Check sheet for the modelled part. Datum: model origin and axes. Units: mm. A direction names the side the tool comes from. Round coordinates to 2 decimals unless told otherwise and drop trailing zeros. Order: outer loops, then holes, each group sorted by start corner. A loop starts at its lowest first (then second) coordinate and runs counter-clockwise, first axis right, second up.
(1) Sectioned sample at C-C, the plane y = 10.5. Enter the section's corners in (x, z), and give its area (3 significant figures).
(2) Sectioned sample at A-A, the plane x = -150. Enter the section's corners in (y, z), and give its area (3 significant figures).
(3) Depth check by flat-ended pin: pin 1 (1.5 mm diameter, centred on x = -39.5, y = 13, fed in from -Z); pin 2 (3 mm diameter, centred on y = 47, z = -23.5, fed in from -X); pin 3 (2 mm diameter, centred on x = -1.5, y = 14, fed in from +Z). Enter the tip coordinate at first touch or a pass-through.
(4) Thickness scan on probe 1 along X at (y, z) = (26, 0); probe 2 along X at (y, z) = (39, 8.5); probe 3 along Y at (x, z) = (126.5, -25). Record the ranges inside material, lowest first.
(5) Sectioned sample at B-B, the plane z = 0. Enter the section's corners in (x, y), and give its area (3 significant figures).
(6) Mould release check, pull along Z, two halves, no side actions. Record for faces 6 (the cylindrical face through (15.02, 34.51, 47.69)), 7 (the cylindrical face through (90.44, 9.86, 36.97)), 8 (the flat face through (45, 70, -23)): released by +Z, released by -Z, zero draft, split by the parting line, or undercut.
(7) Sectioned sample at D-D, the plane x = 0. Enter the section's corners in (y, z), and give its area (3 significant figures).
(8) Tool access check on faces 1 (the cylindrical face through (-91.77, 9.86, 36.69)), 2 (the flat face through (163, 40, -22)), 3 (the flat face through (-138.447, 40, 22.344)), 4 (the cylindrical face through (-90.44, 9.86, -36.97)), 5 (the flat face through (-33, 20, -51)). Record the directions out of +Z, -Z, +X, -X, +Y, -Y that give a thin tool (end or side, any length) a straight path to the whole face; none if there is none.
```python
from build123d import *
from build123d.topology import SkipClean

# Parameters (mm, degrees)
SKETCH1_R           = 60
SKETCH1_R_2         = 25
BOSS_EXTRUDE2_DEPTH = 20
SKETCH1_7_R         = 60
SKETCH1_7_R_2       = 50
BOSS_EXTRUDE3_DEPTH = 70
SKETCH3_R           = 40
SKETCH3_R_2         = 25
BOSS_EXTRUDE4_DEPTH = 20


with BuildPart() as part:
    # Sketch1 → Boss-Extrude2 (new body)
    with BuildSketch(Plane(origin=(0, 0, 0), x_dir=(1, 0, 0), z_dir=(0, 1, 0))):
        with BuildLine():
            ThreePointArc((-139.071428571, 38.478127898), (-190, 0), (-139.071428571, -38.478127898))
            ThreePointArc((-139.071428571, -38.478127898), (-91.104177178, -36.827906099), (-47.892857143, -57.717191847))
            ThreePointArc((-47.892857143, -57.717191847), (0, -75), (47.892857143, -57.717191847))
            ThreePointArc((47.892857143, -57.717191847), (91.104177178, -36.827906099), (139.071428571, -38.478127898))
            ThreePointArc((139.071428571, -38.478127898), (190, 0), (139.071428571, 38.478127898))
            ThreePointArc((139.071428571, 38.478127898), (91.104177178, 36.827906099), (47.892857143, 57.717191847))
            ThreePointArc((47.892857143, 57.717191847), (0, 75), (-47.892857143, 57.717191847))
            ThreePointArc((-47.892857143, 57.717191847), (-91.104177178, 36.827906099), (-139.071428571, 38.478127898))
        make_face()
        with Locations(Location((0, 0, 0), (0, 0, 270))):
            Circle(SKETCH1_R, mode=Mode.SUBTRACT)
        with Locations(Location((-150, 0, 0), (0, 0, 270))):
            Circle(SKETCH1_R_2, mode=Mode.SUBTRACT)
        with Locations(Location((150, 0, 0), (0, 0, 90))):
            Circle(SKETCH1_R_2, mode=Mode.SUBTRACT)
    extrude(amount=BOSS_EXTRUDE2_DEPTH)

    # Sketch1_7 → Boss-Extrude3 (add)
    with BuildSketch(Plane(origin=(0, 0, 0), x_dir=(1, 0, 0), z_dir=(0, 1, 0))):
        with Locations(Location((0, 0, 0), (0, 0, 270))):
            Circle(SKETCH1_7_R)
        with Locations(Location((0, 0, 0), (0, 0, 270))):
            Circle(SKETCH1_7_R_2, mode=Mode.SUBTRACT)
    extrude(amount=BOSS_EXTRUDE3_DEPTH)

    # Sketch3 → Boss-Extrude4 (add)
    with BuildSketch(Plane(origin=(0, 20, 0), x_dir=(1, 0, 0), z_dir=(0, 1, 0))):
        with Locations(Location((-150, 0, 0), (0, 0, 74.144374523))):
            Circle(SKETCH3_R)
        with Locations(Location((-150, 0, 0), (0, 0, 270))):
            Circle(SKETCH3_R_2, mode=Mode.SUBTRACT)
    boss_extrude4 = extrude(amount=BOSS_EXTRUDE4_DEPTH)

    # Mirror1: Boss-Extrude4 across plane
    with SkipClean():  # the faces are left unmerged after this step: merging them gives an invalid solid
        add(boss_extrude4.mirror(Plane(origin=(0, 0, 0), x_dir=(0, 0, 1), z_dir=(1, 0, 0))))


solid = part.part
```
Derived:
1. outline: (-139.07, -38.48) arc R100 cw to (-47.89, -57.72) arc R75 ccw to (47.89, -57.72) arc R100 cw to (139.07, -38.48) arc R40 ccw (long way) to (139.07, 38.48) arc R100 cw to (47.89, 57.72) arc R75 ccw to (-47.89, 57.72) arc R100 cw to (-139.07, 38.48) arc R40 ccw (long way) to start; hole circle Ø50 at (-150, 0); hole circle Ø100 at (0, 0); hole circle Ø50 at (150, 0)
1. area: 22,900 mm2
2. outline: (0, -40) - (40, -40) - (40, -25) - (0, -25) - close; (0, 25) - (40, 25) - (40, 40) - (0, 40) - close
2. area: 1,200 mm2
3. pin 1: stops at z = -64.21
3. pin 2: stops at x = -55.82
3. pin 3: stops at z = 75
4. probe 1: x = -190 to -175, -125 to -110, -60 to -50, 50 to 60, 110 to 125, 175 to 190
4. probe 2: x = -189.09 to -173.51, -126.49 to -110.91, -59.39 to -49.27, 49.27 to 59.39, 110.91 to 126.49, 173.51 to 189.09
4. probe 3: y = 0 to 40
5. outline: (-190, 0) - (-175, 0) - (-175, 40) - (-190, 40) - close; (-125, 0) - (-50, 0) - (-50, 70) - (-60, 70) - (-60, 20) - (-110, 20) - (-110, 40) - (-125, 40) - close; (50, 0) - (125, 0) - (125, 40) - (110, 40) - (110, 20) - (60, 20) - (60, 70) - (50, 70) - close; (175, 0) - (190, 0) - (190, 40) - (175, 40) - close
5. area: 5,800 mm2
6. face 6: undercut
6. face 7: released by +Z
6. face 8: zero draft
7. outline: (0, -75) - (20, -75) - (20, -60) - (70, -60) - (70, -50) - (0, -50) - close; (0, 50) - (70, 50) - (70, 60) - (20, 60) - (20, 75) - (0, 75) - close
7. area: 2,000 mm2
8. face 1: +Z, +Y, -Y
8. face 2: +Z, -Z, +X, +Y
8. face 3: +Z, -Z, -X, +Y
8. face 4: -Z, +Y, -Y
8. face 5: +Y
